CAD build for the part. Positions are in the model's coordinates, mm. A direction names the side the tool comes from. Coordinates: 2 decimals unless noted, no trailing zeros. Loops run counter-clockwise (first coordinate to the right, second up) from the corner with the lowest first, then second, coordinate; pieces in that order, holes last. Notation, with made-up numbers: (-28, -6) -> (4, -6) arc R31 ccw to (4, 23) -> close; hole circle Ø8 at (-35.5, 85). An arc over 180 degrees is marked (long way). Write each question's results on one line, items separated by ' | '.
from build123d import *

# Parameters (mm, degrees)
PAD_DEPTH           = 710
HOLE_D              = 3.4
HOLE_CBORE_D        = 4.8
HOLE_CBORE_DEPTH    = 1.5
HOLE003_D           = 3.4
HOLE003_CBORE_D     = 4.8
HOLE003_CBORE_DEPTH = 1.5
SKETCH006_R         = 12
POCKET_DEPTH        = 12.001
SKETCH008_R         = 1.5
POCKET001_DEPTH     = 8.501
HOLE004_D           = 3.3
HOLE004_DEPTH       = 10
HOLE004_CBORE_D     = 5.5
HOLE004_CBORE_DEPTH = 1
HOLE004_TIPS_R      = 1.65
POCKET003_DEPTH     = 47.001
SKETCH013_W         = 38.5
SKETCH013_H         = 41.5
PAD001_DEPTH        = 10
SKETCH014_R         = 1.65
HOLE005_DEPTH       = 15
HOLE005_TIPS_R      = 1.65
SKETCH015_R         = 1.7
HOLE006_DEPTH       = 50.007254
SKETCH016_R         = 7
POCKET005_DEPTH     = 3
POCKET006_DEPTH     = 47.007254
SKETCH018_R         = 1.7
HOLE007_DEPTH       = 47.007254
SKETCH012_R         = 1.7
HOLE008_DEPTH       = 8.501
SKETCH019_R         = 7
POCKET007_DEPTH     = 3


with BuildPart() as part:
    # Sketch → Pad (new body)
    with BuildSketch(Plane.XZ):
        Polygon((0.045854, -0.006254), (0.045854, 44.993746), (-6.954146, 44.993746), (-6.954146, 49.993746), (5.045854, 49.993746), (5.045854, 8.493746), (43.545854, 8.493746), (43.545854, -0.006254), align=None)
    extrude(amount=PAD_DEPTH)

    # Hole (through all)
    with Locations(Plane(origin=(0, 0, 49.993746), x_dir=(-1, 0, 0), z_dir=(0, 0, 1))):
        with Locations((3.5, 85), (3.5, 635)):
            CounterBoreHole(HOLE_D / 2, HOLE_CBORE_D / 2, HOLE_CBORE_DEPTH)

    # Hole003 (through all)
    with Locations(Plane(origin=(0, 0, 49.993746), x_dir=(-1, 0, 0), z_dir=(0, 0, 1))):
        with Locations((3.5, 375)):
            CounterBoreHole(HOLE003_D / 2, HOLE003_CBORE_D / 2, HOLE003_CBORE_DEPTH)

    # Sketch006 → Pocket (cut, through all)
    with BuildSketch(Plane(origin=(5.045854, 0, 0), x_dir=(0, 0, 1), z_dir=(1, 0, 0))):
        with Locations((29.25, 55)):
            Circle(SKETCH006_R)
    extrude(amount=-POCKET_DEPTH, mode=Mode.SUBTRACT)

    # Sketch008 → Pocket001 (cut, through all)
    with BuildSketch(Plane(origin=(0, 0, 8.493746), x_dir=(-1, 0, 0), z_dir=(0, 0, 1))):
        with Locations((-34.25, 55)):
            Circle(SKETCH008_R)
        with Locations((-12.25, 55)):
            Circle(SKETCH008_R)
    extrude(amount=-POCKET001_DEPTH, mode=Mode.SUBTRACT)

    # Hole004
    with Locations(Plane(origin=(0, 0, -0.006254), x_dir=(1, 0, 0), z_dir=(0, 0, -1))):
        with Locations((12.25, 5), (34.25, 5)):
            CounterBoreHole(HOLE004_D / 2, HOLE004_CBORE_D / 2, HOLE004_CBORE_DEPTH, depth=HOLE004_DEPTH)

    # Hole004 tips → Hole004 tip 1 section 0
    with BuildSketch(Plane(origin=(0, 0, 9.993746), x_dir=(1, 0, 0), z_dir=(0, 0, -1)), mode=Mode.PRIVATE) as hole004_tip_1_s0:
        with Locations((12.25, 5)):
            Circle(HOLE004_TIPS_R)
    loft([hole004_tip_1_s0.sketch, Vertex(12.25, -5, 10.985166)], mode=Mode.SUBTRACT)

    # Hole004 tips → Hole004 tip 2 section 0
    with BuildSketch(Plane(origin=(0, 0, 9.993746), x_dir=(1, 0, 0), z_dir=(0, 0, -1)), mode=Mode.PRIVATE) as hole004_tip_2_s0:
        with Locations((34.25, 5)):
            Circle(HOLE004_TIPS_R)
    loft([hole004_tip_2_s0.sketch, Vertex(34.25, -5, 10.985166)], mode=Mode.SUBTRACT)

    # Sketch011 → Pocket003 (cut, through all)
    with BuildSketch(Plane(origin=(0, 0, 2.993746), x_dir=(1, 0, 0), z_dir=(0, 0, -1))):
        with BuildLine():
            ThreePointArc((21, 56.2), (19.8, 55), (21, 53.8))
            Line((21, 53.8), (26, 53.8))
            ThreePointArc((26, 53.8), (27.2, 55), (26, 56.2))
            Line((26, 56.2), (21, 56.2))
        make_face()
    extrude(amount=-POCKET003_DEPTH, mode=Mode.SUBTRACT)

    # Sketch013 → Pad001 (join)
    with BuildSketch(Plane(origin=(0, 0, 0), x_dir=(1, 0, 0), z_dir=(0, 1, 0))):
        with Locations((24.25, -29.25)):
            Rectangle(SKETCH013_W, SKETCH013_H)
    extrude(amount=-PAD001_DEPTH)

    # Sketch014 → Hole005 (cut)
    with BuildSketch(Plane(origin=(0, 0, 8.5), x_dir=(1, 0, 0), z_dir=(0, 0, -1))):
        with Locations((12.25, 5)):
            Circle(SKETCH014_R)
        with Locations((34.25, 5)):
            Circle(SKETCH014_R)
    extrude(amount=-HOLE005_DEPTH, mode=Mode.SUBTRACT)

    # Hole005 tips → Hole005 tip 1 section 0
    with BuildSketch(Plane(origin=(0, 0, 23.5), x_dir=(1, 0, 0), z_dir=(0, 0, -1)), mode=Mode.PRIVATE) as hole005_tip_1_s0:
        with Locations((12.25, 5)):
            Circle(HOLE005_TIPS_R)
    loft([hole005_tip_1_s0.sketch, Vertex(12.25, -5, 24.49142)], mode=Mode.SUBTRACT)

    # Hole005 tips → Hole005 tip 2 section 0
    with BuildSketch(Plane(origin=(0, 0, 23.5), x_dir=(1, 0, 0), z_dir=(0, 0, -1)), mode=Mode.PRIVATE) as hole005_tip_2_s0:
        with Locations((34.25, 5)):
            Circle(HOLE005_TIPS_R)
    loft([hole005_tip_2_s0.sketch, Vertex(34.25, -5, 24.49142)], mode=Mode.SUBTRACT)

    # Sketch015 → Hole006 (cut, through all)
    with BuildSketch(Plane(origin=(0, 0, -0.006254), x_dir=(1, 0, 0), z_dir=(0, 0, -1))):
        with Locations((12.25, 575)):
            Circle(SKETCH015_R)
        with Locations((34.25, 575)):
            Circle(SKETCH015_R)
    extrude(amount=-HOLE006_DEPTH, mode=Mode.SUBTRACT)

    # Sketch016 → Pocket005 (cut)
    with BuildSketch(Plane(origin=(0, 0, -0.006254), x_dir=(1, 0, 0), z_dir=(0, 0, -1))):
        with Locations((23.5, 575)):
            Circle(SKETCH016_R)
    extrude(amount=-POCKET005_DEPTH, mode=Mode.SUBTRACT)

    # Sketch017 → Pocket006 (cut, through all)
    with BuildSketch(Plane(origin=(0, 0, 2.993746), x_dir=(1, 0, 0), z_dir=(0, 0, -1))):
        with BuildLine():
            ThreePointArc((21, 576.2), (19.8, 575), (21, 573.8))
            Line((21, 573.8), (26, 573.8))
            ThreePointArc((26, 573.8), (27.2, 575), (26, 576.2))
            Line((26, 576.2), (21, 576.2))
        make_face()
    extrude(amount=-POCKET006_DEPTH, mode=Mode.SUBTRACT)

    # Sketch018 → Hole007 (cut, through all)
    with BuildSketch(Plane(origin=(0, 0, 2.993746), x_dir=(1, 0, 0), z_dir=(0, 0, -1))):
        with Locations((21, 575)):
            Circle(SKETCH018_R)
        with Locations((26, 575)):
            Circle(SKETCH018_R)
    extrude(amount=-HOLE007_DEPTH, mode=Mode.SUBTRACT)

    # Sketch012 (on Face15 of Pocket003) → Hole008 (cut, through all)
    with BuildSketch(Plane(origin=(0, 0, 8.493746), x_dir=(-1, 0, 0), z_dir=(0, 0, 1))):
        with Locations((-21, 55)):
            Circle(SKETCH012_R)
        with Locations((-26, 55)):
            Circle(SKETCH012_R)
    extrude(amount=-HOLE008_DEPTH, mode=Mode.SUBTRACT)

    # Sketch019 → Pocket007 (cut)
    with BuildSketch(Plane(origin=(0, 0, -0.006254), x_dir=(1, 0, 0), z_dir=(0, 0, -1))):
        with Locations((23.5, 55)):
            Circle(SKETCH019_R)
    extrude(amount=-POCKET007_DEPTH, mode=Mode.SUBTRACT)


solid = part.part
1) Two-plate mould, pull along X, no slides. Class faces 4 (the flat face through (0.046, -350, 22)), 5 (the cylindrical face through (22.59, -61.94, 1.47)), 6 (the flat face through (22, -350, -0.006)): pulls with the +X half, pulls with the -X half, needs draft (parallel to the pull), parting line crosses it, or undercut.
Outcome:
face 4: pulls with the -X half | face 5: undercut | face 6: needs draft
2) Slice it at A-A (z = 35.5). Write the cut outline in (x, y), then the cut area to 3 significant figures.
Outcome:
outline: (0.05, -710) -> (5.05, -710) -> (5.05, -65.24) -> (0.05, -65.24) -> close; (0.05, -44.76) -> (5.05, -44.76) -> (5.05, -10) -> (43.5, -10) -> (43.5, 0) -> (0.05, 0) -> close | area: 3,830 mm^2
3) Pin check, flat tips, straight feed: pin 1 (2 mm diameter, centred on x = 12.25, y = -575, fed in from -Z); pin 2 (10 mm diameter, centred on x = 2.5, y = -536, fed in from +Z); pin 3 (4 mm diameter, centred on y = -456.5, z = 15, fed in from -X); pin 4 (6 mm diameter, centred on x = 18.5, y = -533.5, fed in from +Z). Stop position of each tip, or through.
Outcome:
pin 1: passes through | pin 2: stops at z = 49.99 | pin 3: stops at x = 0.05 | pin 4: stops at z = 8.49
4) Drill centre lines: L1, parallel to Y at x = -3.5, z = 46.6; L2, parallel to Y at x = 12.25, z = 3.25; L3, parallel to X at y = -375, z = 49.1. Where is each one in solid material? Low to high. Write a range as from..to.
Outcome:
L1: y = -710..-636.7, -633.3..-376.7, -373.3..-86.7, -83.3..0 | L2: y = -710..-576.7, -573.3..-56.5, -53.5..-6.65, -3.35..0 | L3: x = -6.95..-5.9, -1.1..5.05
5) Which spindle directions (+Z, -Z, +X, -X, +Y, -Y) get a long thin tool onto all of the face, cutting with end or side? Do faces 1 (the cylindrical face through (18.34, -579.73, 1.47)), 2 (the flat face through (24, -10, 29)), 3 (the flat face through (17, -710, 8)). Say none if no direction does.
Outcome:
face 1: -Z | face 2: +Z, +X, -Y | face 3: +Z, -Z, +X, -X, -Y
